```python
from build123d import *

# Parameters (mm, degrees)
SKETCH1_W           = 170
SKETCH1_H           = 163.12
SKETCH1_R           = 5
BOSS_EXTRUDE1_DEPTH = 6.35


with BuildPart() as part:
    # Sketch1 → Boss-Extrude1 (new body)
    with BuildSketch(Plane.XY):
        with Locations((85, 81.56)):
            Rectangle(SKETCH1_W, SKETCH1_H)
        with Locations((85, 7)):
            Circle(SKETCH1_R, mode=Mode.SUBTRACT)
        with Locations((152, 7)):
            Circle(SKETCH1_R, mode=Mode.SUBTRACT)
        with Locations((18, 7)):
            Circle(SKETCH1_R, mode=Mode.SUBTRACT)
        with Locations((18, 81.56)):
            Circle(SKETCH1_R, mode=Mode.SUBTRACT)
        with Locations((18, 156.12)):
            Circle(SKETCH1_R, mode=Mode.SUBTRACT)
        with Locations((152, 81.56)):
            Circle(SKETCH1_R, mode=Mode.SUBTRACT)
        with Locations((152, 156.12)):
            Circle(SKETCH1_R, mode=Mode.SUBTRACT)
        with Locations((85, 156.12)):
            Circle(SKETCH1_R, mode=Mode.SUBTRACT)
    extrude(amount=-BOSS_EXTRUDE1_DEPTH)


solid = part.part
```
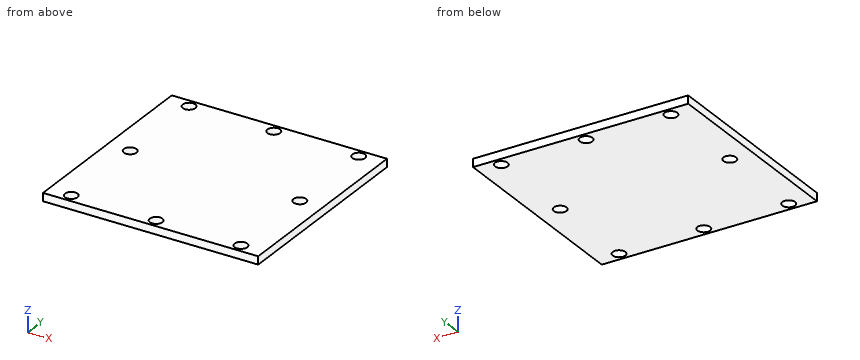
CAD build for the part. Positions are in the model's coordinates, mm. Coordinates: 2 decimals unless noted, no trailing zeros. Loops run counter-clockwise (first coordinate to the right, second up) from the corner with the lowest first, then second, coordinate; pieces in that order, holes last. Notation, with made-up numbers: (28.25, 68.25) - (87.25, 68.25) arc R36 cw to (87.25, 105.25) - close; hole circle Ø5 at (-33, -36). An arc over 180 degrees is marked (long way). Return JSON: item names as keys, results as strings.
1. Band-saw the part on B-B (y = 81.56). Give the cut face in (x, z), and give its area (4 significant figures).
Result:
{"outline": "(0, -6.35) - (13, -6.35) - (13, 0) - (0, 0) - close; (23, -6.35) - (147, -6.35) - (147, 0) - (23, 0) - close; (157, -6.35) - (170, -6.35) - (170, 0) - (157, 0) - close", "area": "952.5 mm2"}
2. Band-saw the part on C-C (z = -1). State how many separate pieces and enclosed holes the cut face has, and give its area (3 significant figures).
Result:
{"separate pieces": "1", "enclosed holes": "8", "area": "27,100 mm2"}
3. Band-saw the part on D-D (x = 85). Give the cut face in (y, z), and give its area (3 significant figures).
Result:
{"outline": "(0, -6.35) - (2, -6.35) - (2, 0) - (0, 0) - close; (12, -6.35) - (151.12, -6.35) - (151.12, 0) - (12, 0) - close; (161.12, -6.35) - (163.12, -6.35) - (163.12, 0) - (161.12, 0) - close", "area": "909 mm2"}
4. Band-saw the part on A-A (x = 152). Give the cut face in (y, z), and give its area (3 significant figures).
Result:
{"outline": "(0, -6.35) - (2, -6.35) - (2, 0) - (0, 0) - close; (12, -6.35) - (76.56, -6.35) - (76.56, 0) - (12, 0) - close; (86.56, -6.35) - (151.12, -6.35) - (151.12, 0) - (86.56, 0) - close; (161.12, -6.35) - (163.12, -6.35) - (163.12, 0) - (161.12, 0) - close", "area": "845 mm2"}
5. Drop a flat-ended pin along its axis: pin 1 (8 mm diameter, centred on x = 152, y = 156.12, fed in from +Z). Give the stop position or say it passes through.
Result:
{"pin 1": "passes through"}
6. Probe L1, parallel to Y at x = 152, z = -2; L2, parallel to Y at x = 85, z = -3.25; L3, parallel to X at y = 81.5, z = -2.75. List the from-to ranges inside material, lowest first. Write a range as from..to.
Result:
{"L1": "y = 0..2, 12..76.56, 86.56..151.12, 161.12..163.12", "L2": "y = 0..2, 12..151.12, 161.12..163.12", "L3": "x = 0..13, 23..147, 157..170"}
